```python
from build123d import *

# Parameters (mm, degrees)
SKETCH1_W           = 8.3
SKETCH1_H           = 24.8
SKETCH1_W_2         = 125.2
SKETCH1_H_2         = 7.3
SKETCH1_W_3         = 11.1
SKETCH1_H_3         = 42.4
BOSS_EXTRUDE1_DEPTH = 153.4
SKETCH2_R           = 3
CUT_EXTRUDE1_DEPTH  = 153.4
LPATTERN1_COUNT     = 2
LPATTERN1_PITCH     = 100


with BuildPart() as part:
    # Sketch1 → Boss-Extrude1 (new body)
    with BuildSketch(Plane.XY):
        with Locations((-58.45, 16.05)):
            Rectangle(SKETCH1_W, SKETCH1_H)
        Rectangle(SKETCH1_W_2, SKETCH1_H_2)
        with Locations((16.35, 24.85)):
            Rectangle(SKETCH1_W_3, SKETCH1_H_3)
    extrude(amount=BOSS_EXTRUDE1_DEPTH)

    # Sketch2 → Cut-Extrude1 (cut)
    with BuildSketch(Plane(origin=(0, 3.65, 0), x_dir=(1, 0, 0), z_dir=(0, 1, 0))):
        with Locations(Location((45, -25, 0), (0, 0, 270))):
            Circle(SKETCH2_R)
    cut_extrude1 = extrude(amount=-CUT_EXTRUDE1_DEPTH, mode=Mode.SUBTRACT)

    # LPattern1: Cut-Extrude1 ×2
    with Locations(*[(0, 0, i * LPATTERN1_PITCH) for i in range(1, LPATTERN1_COUNT)]):
        add(cut_extrude1, mode=Mode.SUBTRACT)


solid = part.part
```
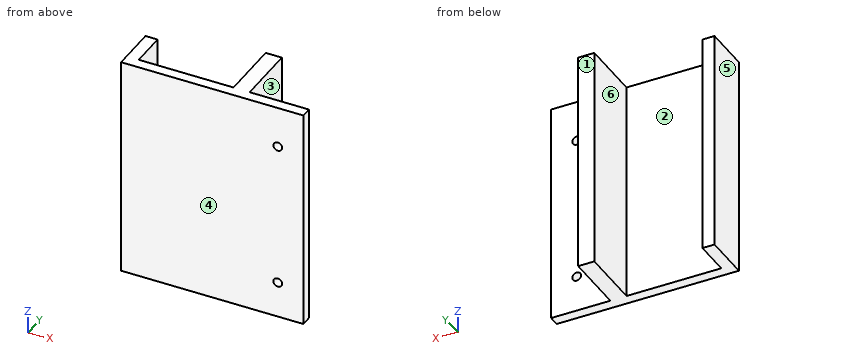
Could you check a few things on this model? Use its own coordinates, in mm. Face numbers are marked on the shaded views. A direction names the side the tool comes from. Round coordinates to 2 decimals unless told otherwise and drop trailing zeros. Write each loop counter-clockwise with the first axis right and the second up, starting at its lowest first coordinate (ties: lowest second). Pieces come first, ordered by that corner, then holes. Notation, with made-up numbers: M 62.25,71.5 L 76.25,71.5 A29 ccw 76.25,106.5 Z; hole C -39.75,-4 d5. An arc over 180 degrees is marked long. Answer in a Markdown table with one row per item. Add a question column.
Q1. Will these pins go through, and if not, where does the flat tip stop? pin 1 Ø2.5 at (x, z) = (-60, 59.5) entering from +Y; pin 2 Ø12 at (x, z) = (-2.5, 22) entering from +Y; pin 3 Ø7 at (x, z) = (45, 125) entering from +Y; pin 4 Ø3.5 at (x, z) = (45, 25) entering from +Y.
Q2. On a 3-axis mill with a long thin cutter (end or side, diameter ignored), from which of +Z, -Z, +X, -X, +Y, -Y can I reach the whole of each face in a straight line? I mean the marked faces 1, 2 and 3. Say none if no direction works.
Q3. If we mould it in two halves opening along X, with no side actions, what happens to the marked faces 4, 5 and 6? For each: +X half, -X half, draft (parallel to the pull), parting line (faces both ways), or undercut.
Q4. If I drill on line 1 (X direction, y = 21, z = 48); line 2 (Y direction, x = 52, z = 102.5); line 3 (X direction, y = 39, z = 118), over which ranges is the centre line in solid material (lowest first)? Write a range as from..to.
Q5. Imagine slicing it at B-B (z = 25). Please give me the cut outline in (x, y).
Q6. Imagine slicing it at C-C (x = 45). Please give me the cut outline in (y, z).
Q7. Imagine slicing it at D-D (z = 81). Please give me the cut outline in (x, y).
Q8. Imagine slicing it at A-A (y = 23.5). Please give me the cut outline in (x, z).
Values:
| question | item | result |
|---|---|---|
| 1 | pin 1 | y = 28.45 |
| 1 | pin 2 | y = 3.65 |
| 1 | pin 3 | y = 3.65 |
| 1 | pin 4 | through |
| 2 | face 1 | +Z, -Z, +X, -X, +Y |
| 2 | face 2 | +Z, -Z, +Y |
| 2 | face 3 | +Z, -Z, +X, +Y |
| 3 | face 4 | draft |
| 3 | face 5 | -X half |
| 3 | face 6 | undercut |
| 4 | line 1 | -62.6..-54.3, 10.8..21.9 |
| 4 | line 2 | -3.65..3.65 |
| 4 | line 3 | 10.8..21.9 |
| 5 | outline | M -62.6,-3.65 L 42,-3.65 L 42,3.65 L 21.9,3.65 L 21.9,46.05 L 10.8,46.05 L 10.8,3.65 L -54.3,3.65 L -54.3,28.45 L -62.6,28.45 Z; M 48,-3.65 L 62.6,-3.65 L 62.6,3.65 L 48,3.65 Z |
| 6 | outline | M -3.65,0 L 3.65,0 L 3.65,22 L -3.65,22 Z; M -3.65,28 L 3.65,28 L 3.65,122 L -3.65,122 Z; M -3.65,128 L 3.65,128 L 3.65,153.4 L -3.65,153.4 Z |
| 7 | outline | M -62.6,-3.65 L 62.6,-3.65 L 62.6,3.65 L 21.9,3.65 L 21.9,46.05 L 10.8,46.05 L 10.8,3.65 L -54.3,3.65 L -54.3,28.45 L -62.6,28.45 Z |
| 8 | outline | M -62.6,0 L -54.3,0 L -54.3,153.4 L -62.6,153.4 Z; M 10.8,0 L 21.9,0 L 21.9,153.4 L 10.8,153.4 Z |
